```python
from build123d import *

# Parameters (mm, degrees)
SKETCH1_W           = 96
SKETCH1_H           = 89
BOSS_EXTRUDE1_DEPTH = 72.5
SKETCH3_W           = 91
SKETCH3_H           = 84
CUT_EXTRUDE1_DEPTH  = 70
CUT_EXTRUDE5_DEPTH  = 90
SKETCH7_R           = 3.75
SKETCH7_R_2         = 5
CUT_EXTRUDE6_DEPTH  = 2.5
SKETCH8_W           = 42
SKETCH8_H           = 21.66
CUT_EXTRUDE7_DEPTH  = 2.5
CUT_EXTRUDE8_DEPTH  = 2.5
FILLET1_R           = 2.5


with BuildPart() as part:
    # Sketch1 → Boss-Extrude1 (new body)
    with BuildSketch(Plane(origin=(0, 0, 0), x_dir=(1, 0, 0), z_dir=(0, 1, 0))):
        with Locations((48, -44.5)):
            Rectangle(SKETCH1_W, SKETCH1_H)
    extrude(amount=BOSS_EXTRUDE1_DEPTH)

    # Sketch3 → Cut-Extrude1 (cut)
    with BuildSketch(Plane(origin=(0, 72.5, 0), x_dir=(1, 0, 0), z_dir=(0, 1, 0))):
        with Locations((48, -44.5)):
            Rectangle(SKETCH3_W, SKETCH3_H)
    extrude(amount=-CUT_EXTRUDE1_DEPTH, mode=Mode.SUBTRACT)

    # Sketch5 → Cut-Extrude5 (cut, through all)
    with BuildSketch(Plane.XY.offset(89)):
        Polygon((0, 31.16), (0, 72.5), (96, 72.5), (96, 49.95), (80.25, 49.95), (71, 49.95), (71, 31.16), align=None)
    extrude(amount=-CUT_EXTRUDE5_DEPTH, mode=Mode.SUBTRACT)

    # Sketch7 → Cut-Extrude6 (cut)
    with BuildSketch(Plane.XY.offset(89)):
        with Locations((80.25, 49.95)):
            Circle(SKETCH7_R)
        with Locations((60.9, 31.16)):
            Circle(SKETCH7_R_2)
    extrude(amount=-CUT_EXTRUDE6_DEPTH, mode=Mode.SUBTRACT)

    # Sketch8 → Cut-Extrude7 (cut)
    with BuildSketch(Plane(origin=(0, 0, 0), x_dir=(-1, 0, 0), z_dir=(0, 0, -1))):
        with Locations((-50, 20.33)):
            Rectangle(SKETCH8_W, SKETCH8_H)
    extrude(amount=-CUT_EXTRUDE7_DEPTH, mode=Mode.SUBTRACT)

    # Sketch9 → Cut-Extrude8 (cut)
    with BuildSketch(Plane(origin=(0, 0, 0), x_dir=(-1, 0, 0), z_dir=(0, 0, -1))):
        with BuildLine():
            Line((-55, 9.5), (-45, 9.5))
            ThreePointArc((-45, 9.5), (-50, 4.5), (-55, 9.5))
        make_face()
    extrude(amount=-CUT_EXTRUDE8_DEPTH, mode=Mode.SUBTRACT)

    # Fillet1
    fillet1_edges = [part.edges().sort_by_distance(p)[0] for p in [
        (0, 15.58, 0),
        (96, 24.975, 0),
        (96, 24.975, 89),
        (0, 15.58, 89),
        (48, 0, 0),
        (96, 0, 44.5),
        (48, 0, 89),
        (0, 0, 44.5),
    ]]
    fillet(fillet1_edges, radius=FILLET1_R)


solid = part.part
```
For this review, take the finished solid that the model builds, in its own axes (mm). A direction names the side the tool comes from. Round coordinates to 2 decimals unless told otherwise and drop trailing zeros. Write each loop counter-clockwise with the first axis right and the second up, starting at its lowest first coordinate (ties: lowest second). Pieces come first, ordered by that corner, then holes. Notation, with made-up numbers: M 25,15 L 35,15 A16 ccw 35,40 Z; hole C -35.75,22 d6. An arc over 180 degrees is marked long. One line per item, written item: value. Start each with the question number.
(1) We need section C-C (z = 55). Give the boundary of the cut face in (x, y), and give its area (3 significant figures).
(2) Machinability: for faces 1 (the flat face through (47, 0, 44)), 2 (the flat face through (74, 49.95, 88)), 3 (the flat face through (68, 31.16, 88)), 4 (the flat face through (47, 21, 86.5)), 5 (the flat face through (29, 20, 1)), which of the approach directions +Z, -Z, +X, -X, +Y, -Y give a long, thin tool a straight path to every point of the face, cutting with its end or side? Answer none if there is none.
(3) We need section A-A (x = 50). Give the boundary of the cut face in (y, z).
(4) Wall thickness on line 1 (X direction, y = 15.5, z = 47.5); line 2 (Z direction, x = 79, y = 24.5); line 3 (Y direction, x = 21, z = 77): over which ranges is each line inside the solid? List them lowest first.
(5) We need section B-B (y = 14). Give the boundary of the cut face in (x, z).
(6) We need section D-D (y = 6.5). Give the boundary of the cut face in (x, z).
(7) Insertion check: pin 1 (0.8 mm diameter, centred on y = 35.5, z = 1.5, fed in from -X); pin 2 (1.2 mm diameter, centred on x = 40, z = 1, fed in from +Y); pin 3 (1.2 mm diameter, centred on y = 18, z = 1.5, fed in from +X); pin 4 (6 mm diameter, centred on x = 63.5, y = 34.5, fed in from +Z). Each pin has a flat end and moves straight along its axis. Give the tip position at first contact, or say it passes through.
(8) The part is to be moulded in two halves that separate along Z. For faces 6 (the flat face through (2.5, 17, 45)), 7 (the cylindrical face through (49.9, 4.5, 1.2)), 8 (the flat face through (57, 21, 89)), say which applies: released by +Z, released by -Z, zero draft, split by the parting line, or undercut.
Result:
1. outline: M 0,2.5 A2.5 ccw 2.5,0 L 93.5,0 A2.5 ccw 96,2.5 L 96,49.95 L 93.5,49.95 L 93.5,2.5 L 2.5,2.5 L 2.5,31.16 L 0,31.16 Z
1. area: 428 mm²
2. face 1: +Z, -Z, +X, -X, -Y
2. face 2: +Z, -Z, +X, -X, +Y
2. face 3: +Z, -Z, -X, +Y
2. face 4: +Y
2. face 5: -Z, +Y
3. outline: M 0,2.5 A2.5 ccw 2.5,0 L 4.5,0 L 4.5,2.5 L 2.5,2.5 L 2.5,86.5 L 31.16,86.5 L 31.16,89 L 2.5,89 A2.5 ccw 0,86.5 Z
4. line 1: 0 to 2.5, 93.5 to 96
4. line 2: 0 to 2.5, 86.5 to 89
4. line 3: 0 to 2.5
5. outline: M 0,2.5 A2.5 ccw 2.5,0 L 29,0 L 29,2.5 L 2.5,2.5 L 2.5,86.5 L 93.5,86.5 L 93.5,2.5 L 71,2.5 L 71,0 L 93.5,0 A2.5 ccw 96,2.5 L 96,86.5 A2.5 ccw 93.5,89 L 2.5,89 A2.5 ccw 0,86.5 Z
6. outline: M 0,2.5 A2.5 ccw 2.5,0 L 46,0 L 46,2.5 L 2.5,2.5 L 2.5,86.5 L 93.5,86.5 L 93.5,2.5 L 54,2.5 L 54,0 L 93.5,0 A2.5 ccw 96,2.5 L 96,86.5 A2.5 ccw 93.5,89 L 2.5,89 A2.5 ccw 0,86.5 Z
7. pin 1: x = 71
7. pin 2: y = 9.5
7. pin 3: x = 95.97
7. pin 4: through
8. face 6: undercut
8. face 7: zero draft
8. face 8: released by +Z
